Autodesk Inventor part; units mm, degrees
ref_plane "YZ Plane" through (0, 0, 0) normal (1, 0, 0) x (0, 1, 0)
ref_plane "XZ Plane" through (0, 0, 0) normal (0, 1, 0) x (-1, 0, 0)
ref_plane "XY Plane" through (0, 0, 0) normal (0, 0, 1) x (1, 0, 0)
sketch "スケッチ1" plane through (0, 0, 0) normal (0, 0, 1) x (1, 0, 0)
  circle A0 centre (0, 0) radius 2.75
  dimension "d0" = 5.5
extrude "押し出し1" add sketch "スケッチ1" along normal blind 2
sketch "スケッチ2" plane through (0, 0, 0) normal (0, 0, -1) x (-1, 0, 0)
  circle A0 centre (0, 0) radius 2.75
  circle A1 centre (0, 0) radius 1.5
  dimension "d3" = 3
extrude "押し出し2" add sketch "スケッチ2" along normal blind 10 contours A1
sketch "スケッチ3" plane through (0, 0, 2) normal (0, 0, 1) x (1, 0, 0)
  circle A0 centre (0, 0) radius 2.75
  line L0 (0, 1.4434) -> (1.25, 0.7217)
  line L1 (1.25, 0.7217) -> (1.25, -0.7217)
  line L2 (1.25, -0.7217) -> (0, -1.4434)
  line L3 (0, -1.4434) -> (-1.25, -0.7217)
  line L4 (-1.25, -0.7217) -> (-1.25, 0.7217)
  line L5 (-1.25, 0.7217) -> (0, 1.4434)
  dimension "d6" = 1.25
extrude "押し出し3" cut sketch "スケッチ3" against normal blind 1.5 contours L0 L1 L2 L3 L4 L5
fillet "フィレット1" radius 0.3 2 edges at (-2.75, 0, 2) (-2.75, 0, 0)
fillet "フィレット2" radius 0.2 19 edges at (-0.625, 1.0825, 2) (-1.25, 0, 2) (-0.625, -1.0825, 2) (0.625, -1.0825, 2) (1.25, 0, 2) (0.625, 1.0825, 2) (-0.625, 1.0825, 0.5) (0.625, 1.0825, 0.5) (0, 1.4434, 1.25) (-1.25, 0.7217, 1.25) (-0.625, -1.0825, 0.5) (-1.25, -0.7217, 1.25) (-1.25, 0, 0.5) (1.25, 0, 0.5) (1.25, 0.7217, 1.25) (1.25, -0.7217, 1.25) (0.625, -1.0825, 0.5) (0, -1.4434, 1.25) (1.5, 0, -10)
thread "ねじ2"
Source: CAD feature listing. Evaluate the final solid. Frame: model axes, mm. A direction names the side the tool comes from. Give positions to 0.01 mm unless a question says otherwise; leave off trailing zeros. Loops run counter-clockwise (first coordinate to the right, second up) from the corner with the lowest first, then second, coordinate; pieces in that order, holes last. Notation, with made-up numbers: (24.25, 58) - (50.25, 58) arc R16 ccw to (50.25, 63) - close; hole circle Ø9 at (22.25, 15). An arc over 180 degrees is marked (long way). Use CSV: the item, a comma, the result in double quotes. Start each with the question number.
1. Section A-A (y = 0). Output: boundary loops of the cut face in (x, z).
2. Ray query, L1, parallel to Z at x = 0.35, y = 0.8; L2, parallel to Y at x = 0, z = -4.5; L3, parallel to Z at x = 1.1, y = 2.1. Return the intervals inside material, ascending.
3. Draft query along Y for faces 1 (the flat face through (0.618, 1.087, 1.258)), 2 (the flat face through (-0.618, -1.087, 1.258)), 3 (the flat face through (2, 0, 2)), 4 (the cylindrical face through (1.5, -0.07, -4.83)). Return one class per face: +Y half, -Y half, draft (parallel to the pull), parting line (faces both ways), or undercut.
4. Section B-B (z = -8.75). Output: boundary loops of the cut face in (x, y), then the cut area to 3 significant figures.
5. Reachability of faces 5 (the flat face through (0, 0, 0.5)), 6 (the flat face through (0, -2, 0)), 7 (the cylindrical face through (-0.596, 2.685, 0.99)) from +Z, -Z, +X, -X, +Y, -Y: full face, straight path, thin tool, end or side. Return the list, or none.
6. Pin query (flat end, axial travel): pin 1 (1.5 mm diameter, centred on x = 0, y = 1.5, fed in from -Z); pin 2 (3 mm diameter, centred on x = 1, z = -4.5, fed in from -Y); pin 3 (1.7 mm diameter, centred on x = 0, y = 0, fed in from +Z); pin 4 (3 mm diameter, centred on y = 1.5, z = -4, fed in from +X). Return the tip coordinate at first contact, or that it passes through.
Response:
1,outline,"(-2.75, 0.3) arc R0.3 ccw to (-2.45, 0) - (-1.5, 0) - (-1.5, -9.8) arc R0.2 ccw to (-1.3, -10) - (1.3, -10) arc R0.2 ccw to (1.5, -9.8) - (1.5, 0) - (2.45, 0) arc R0.3 ccw to (2.75, 0.3) - (2.75, 1.7) arc R0.3 ccw to (2.45, 2) - (1.45, 2) arc R0.2 ccw to (1.25, 1.8) - (1.25, 0.7) arc R0.2 cw to (1.05, 0.5) - (-1.05, 0.5) arc R0.2 cw to (-1.25, 0.7) - (-1.25, 1.8) arc R0.2 ccw to (-1.45, 2) - (-2.45, 2) arc R0.3 ccw to (-2.75, 1.7) - close"
2,L1,"-10 to 0.5"
2,L2,"-1.5 to 1.5"
2,L3,"0 to 2"
3,face 1,"undercut"
3,face 2,"undercut"
3,face 3,"draft"
3,face 4,"parting line"
4,outline,"circle Ø3 at (0, 0)"
4,area,"7.07 mm²"
5,face 5,"+Z"
5,face 6,"-Z"
5,face 7,"+Z, -Z"
6,pin 1,"z = -10"
6,pin 2,"y = -1.5"
6,pin 3,"z = 0.5"
6,pin 4,"x = 1.5"
